Can you work these out from the model? Positions are in its coordinate system, mm. Give positions to 0.01 mm unless a question says otherwise; leave off trailing zeros. Loops run counter-clockwise (first coordinate to the right, second up) from the corner with the lowest first, then second, coordinate; pieces in that order, holes last. Notation, with made-up numbers: (24.5, 42) -> (56.5, 42) arc R16 cw to (56.5, 66) -> close; hole circle Ø10 at (69.25, 30.5). An arc over 180 degrees is marked (long way). One line per question, with ' | ' between items.
Autodesk Inventor part; units mm, degrees
ref_plane "YZ Plane" through (0, 0, 0) normal (1, 0, 0) x (0, 1, 0)
ref_plane "XZ Plane" through (0, 0, 0) normal (0, 1, 0) x (-1, 0, 0)
ref_plane "XY Plane" through (0, 0, 0) normal (0, 0, 1) x (1, 0, 0)
sketch "Sketch1" plane through (0, 0, 0) normal (0, 1, 0) x (-1, 0, 0)
  line L0 (-20, 42) -> (20, 42)
  line L1 (20, 42) -> (20, -42)
  line L2 (20, -42) -> (-20, -42)
  line L3 (-20, -42) -> (-20, 42)
  point P0 (0, 0)
  dimension "d0" = 40
  dimension "d1" = 84
  dimension "d2" = 20
  dimension "d3" = 42
extrude "Extrusion1" add sketch "Sketch1" along normal blind 3.5
sketch "Sketch3" plane through (20, 0, -42) normal (0, 0, -1) x (-1, 0, 0)
  line L0 (40, 0) -> (40, 3.5)
  line L1 (0, 3.5) -> (40, 3.5)
  line L2 (40, 0) -> (38.5, 0)
  line L3 (38.5, 0) -> (38.5, 3.5)
  line L4 (38.5, 3.5) -> (40, 3.5)
  line L5 (40, 3.5) -> (40, 0)
  line L6 (0, 0) -> (40, 0)
  line L7 (40, 0) -> (38.5, 1.75)
  line L8 (40, 3.5) -> (38.5, 1.75)
  point P0 (20, 0)
  dimension "d10" = 1.5
extrude "Extrusion2" cut sketch "Sketch3" against normal blind 127.5 contours L7 L8 L0
sketch "Sketch4" plane through (0, 3.5, 0) normal (0, 1, 0) x (1, 0, 0)
  point P0 (0, 0)
sketch "Sketch5" plane through (20, 0, 42) normal (0, 0, 1) x (1, 0, 0)
  line L0 (0, 3.5) -> (-40, 3.5)
  line L1 (0, 0) -> (-40, 0)
  line L2 (0, 3.5) -> (-40, 3.5)
  line L3 (-40, 3.5) -> (-40, 0)
  line L4 (-40, 0) -> (0, 0)
  line L5 (0, 0) -> (0, 3.5)
  line L6 (-38.5, 1.75) -> (-40, 0)
  line L7 (-40, 0) -> (-38.5, 1.75)
  line L8 (-38.5, 1.75) -> (-40, 3.5)
  line L9 (-38.5, 1.75) -> (-40, 3.5)
  point P0 (-20, 0)
extrude "Extrusion3" add sketch "Sketch5" along normal blind 36 contours L5 L1 L6 L8 L0
sketch "Sketch6" plane through (0, 3.5, 0) normal (0, 1, 0) x (1, 0, 0)
  point P0 (0, 0)
sketch "Sketch7" plane through (0, 3.5, 0) normal (0, 1, 0) x (1, 0, 0)
  line L0 (-20, 42) -> (-20, -78)
  line L1 (-20, -78) -> (-13, -78)
  line L2 (-13, -78) -> (-13, -72)
  line L3 (-13, -72) -> (-20, -72)
  line L4 (-20, -72) -> (-20, -78)
  line L5 (-20, -78) -> (20, -78)
  line L6 (-20, -72) -> (-18, -72)
  line L7 (-18, -72) -> (-18, -78)
  line L8 (-18, -78) -> (-20, -78)
  line L9 (-20, -78) -> (-20, -72)
  point P0 (0, 0)
  dimension "d15" = 7
  dimension "d16" = 6
extrude "Extrusion4" add sketch "Sketch7" along normal blind 20 contours L3 L2 L1 L7
equation "\"BendRadius\" = Thickness"
equation "\"BendReliefWidth\" = Thickness"
equation "\"BendReliefDepth\" = 0.5 * Thickness"
equation "\"CornerReliefSize\" = 4 * Thickness"
equation "\"MinimumRemnant\" = 2 * Thickness"
equation "\"TransitionRadius\" = BendRadius"
equation "\"JacobiRadiusSize\" = BendRadius"
equation "\"GapSize\" = Thickness"
properties part number "modelGateGate"
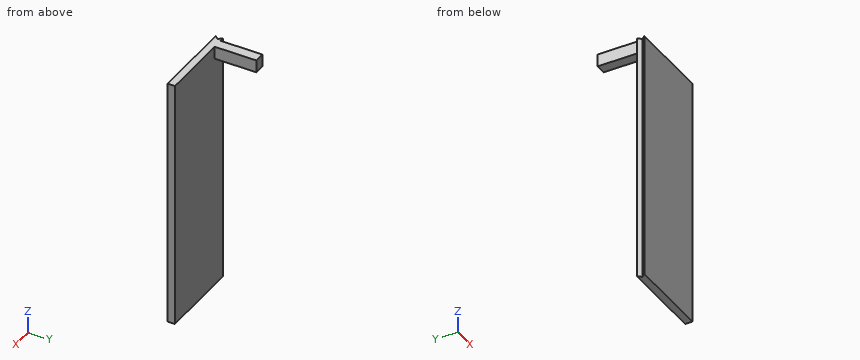
Q1. If we section it at D-D (x = 3.5): Write out the boundary of the cut face in (y, z).
Entries:
outline: (0, -42) -> (3.5, -42) -> (3.5, 78) -> (0, 78) -> close
Q2. If we section it at A-A (z = -7): Write out the boundary of the cut face in (x, y).
Entries:
outline: (-20, 0) -> (20, 0) -> (20, 3.5) -> (-20, 3.5) -> (-18.5, 1.75) -> close
Q3. If we section it at B-B (x = -15): Write out the boundary of the cut face in (y, z), plus the area to 3 significant figures.
Entries:
outline: (0, -42) -> (3.5, -42) -> (3.5, 72) -> (23.5, 72) -> (23.5, 78) -> (0, 78) -> close | area: 540 mm²
Q4. If I drill on probe 1 along Y at (x, z) = (-5.5, -13); probe 2 along Z at (x, y) = (-13.5, 11.5); probe 3 along X at (y, z) = (1, -28.5), over which ranges is the centre line in solid material (lowest first)? Write a range as from..to.
Entries:
probe 1: 0..3.5 | probe 2: 72..78 | probe 3: -19.14..20
Q5. If we section it at C-C (y = 15.25): Write out the boundary of the cut face in (x, z).
Entries:
outline: (-18, 72) -> (-13, 72) -> (-13, 78) -> (-18, 78) -> close
Q6. For pin 1 Ø3 at (y, z) = (15, 76.5) entering from +X; pin 2 Ø3 at (x, z) = (-12.5, 47) entering from -Y; pin 3 Ø4 at (x, y) = (-15.5, 16) entering from -Z; pin 4 Ø5 at (y, z) = (13, 73.5) entering from -X, each with a flat end and sliding along its axis, tell me the tip position at first contact or that it passes through.
Entries:
pin 1: x = -13 | pin 2: y = 0 | pin 3: z = 72 | pin 4: x = -18
